The model under review builds one solid part; all positions refer to its coordinate system, in mm. Coordinates: 2 decimals unless noted, no trailing zeros. Write each loop counter-clockwise with the first axis right and the second up, starting at its lowest first coordinate (ties: lowest second). Pieces come first, ordered by that corner, then holes. Notation, with made-up numbers: M 79,-39.5 L 127,-39.5 A21 cw 127,-18.5 Z; hole C 73,-22 d10. An arc over 180 degrees is marked long. Answer as CSV lines item,"result". Start each with the question number.
Autodesk Inventor part; units mm, degrees
ref_plane "YZ Plane" through (0, 0, 0) normal (1, 0, 0) x (0, 1, 0)
ref_plane "XZ Plane" through (0, 0, 0) normal (0, 1, 0) x (-1, 0, 0)
ref_plane "XY Plane" through (0, 0, 0) normal (0, 0, 1) x (1, 0, 0)
sketch "Sketch1" plane through (0, 0, 0) normal (0, 1, 0) x (-1, 0, 0)
  arc A0 (-3.2658, -7.0635) -> (4, -4.7538) centre (0, -4.7538) ccw
  arc A1 (-4, -4.7538) -> (-3.2658, -7.0635) centre (0, -4.7538) ccw
  line L0 (4, -4.7538) -> (4, 13.2462)
  line L1 (4, 13.2462) -> (8, 13.2462)
  line L2 (10, 15.2462) -> (10, 27.2462)
  line L3 (8, 29.2462) -> (-8, 29.2462)
  line L4 (-10, 27.2462) -> (-10, 15.2462)
  line L5 (-8, 13.2462) -> (-4, 13.2462)
  line L6 (-4, 13.2462) -> (-4, -4.7538)
  circle A2 centre (0, -4.7538) radius 2.65
  arc A3 (8, 13.2462) -> (10, 15.2462) centre (8, 15.2462) ccw
  arc A4 (10, 27.2462) -> (8, 29.2462) centre (8, 27.2462) ccw
  arc A5 (-8, 29.2462) -> (-10, 27.2462) centre (-8, 27.2462) ccw
  arc A6 (-10, 15.2462) -> (-8, 13.2462) centre (-8, 15.2462) ccw
  point P0 (0, 0)
  point P1 (0, 29.2462)
  dimension "d1" = 4
  dimension "d2" = 5.3
  dimension "d6" = 2
  dimension "d7" = 2
  dimension "d9" = 20
  dimension "d10" = 16
  dimension "d13" = 18
extrude "Extrusion2" add sketch "Sketch1" along normal blind 2
properties part number "Pomodoro Robot Servo's piece"
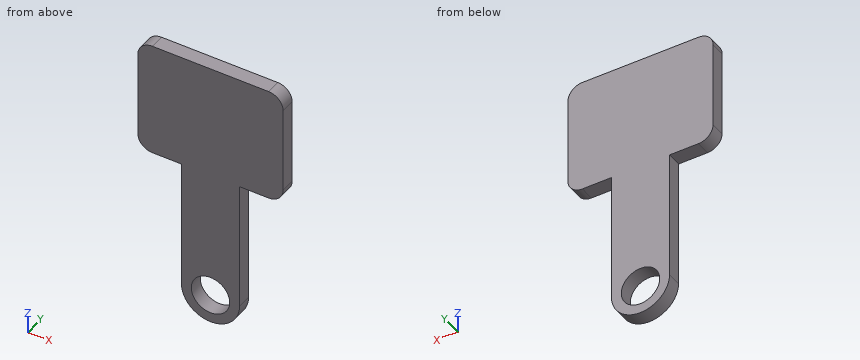
1) Take a section at C-C on z = 0.5. Give the boundary of the cut face in (x, y).
2) Take a section at B-B on x = 0. Give the boundary of the cut face in (y, z).
3) Clearance check with flat-ended pins moving along their axes: pin 1 Ø0.6 at (x, y) = (6.5, 1) entering from -Z; pin 2 Ø0.6 at (y, z) = (0.5, 4.5) entering from +X. State where each tip first meets the part, or that it passes through.
4) Take a section at D-D on x = 4.75. Give the boundary of the cut face in (y, z), and give its area (3 significant figures).
5) To check wall thickness, follow line 1 (Z direction, x = 0, y = 0.65); line 2 (X direction, y = 0.5, z = 10.5); line 3 (Z direction, x = 4.25, y = 1.6). State the ranges of each line that lie inside material, in increasing order. Write a range as [from, to].
6) Take a section at A-A on y = 1.6. Give the boundary of the cut face in (x, z), and give its area (3 significant figures).
Results:
1,outline,"M -4,0 L 4,0 L 4,2 L -4,2 Z"
2,outline,"M 0,-8.75 L 2,-8.75 L 2,-7.4 L 0,-7.4 Z; M 0,-2.1 L 2,-2.1 L 2,29.25 L 0,29.25 Z"
3,pin 1,"stops at z = 13.25"
3,pin 2,"stops at x = 4"
4,outline,"M 0,13.25 L 2,13.25 L 2,29.25 L 0,29.25 Z"
4,area,"32.0 mm²"
5,line 1,"z = [-8.75, -7.4], [-2.1, 29.25]"
5,line 2,"x = [-4, 4]"
5,line 3,"z = [13.25, 29.25]"
6,outline,"M -10,15.25 A2 ccw -8,13.25 L -4,13.25 L -4,-4.75 A4 ccw 3.27,-7.06 A4 ccw 4,-4.75 L 4,13.25 L 8,13.25 A2 ccw 10,15.25 L 10,27.25 A2 ccw 8,29.25 L -8,29.25 A2 ccw -10,27.25 Z; hole C 0,-4.75 d5.3"
6,area,"464 mm²"
